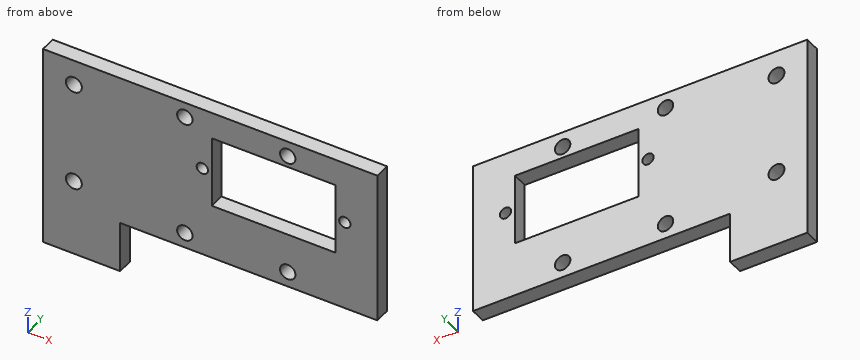
```python
from build123d import *

# Parameters (mm, degrees)
SKETCH_1_W          = 65
SKETCH_1_H          = 40
EXTRUDE_1_DEPTH     = 3
SKETCH_2_R          = 1.55
CUT_EXTRUDE_1_DEPTH = 10
SKETCH_3_W          = 50
SKETCH_3_H          = 10
CUT_EXTRUDE_2_DEPTH = 10
SKETCH_4_W          = 24
SKETCH_4_H          = 14
CUT_EXTRUDE_3_DEPTH = 10
SKETCH_5_R          = 1.1
CUT_EXTRUDE_4_DEPTH = 10
SKETCH_6_R          = 1.5
CUT_EXTRUDE_5_DEPTH = 25


with BuildPart() as part:
    # 草图1 → 凸台-拉伸1 (new body)
    with BuildSketch(Plane(origin=(0, 0, 0), x_dir=(1, 0, 0), z_dir=(0, 1, 0))):
        Rectangle(SKETCH_1_W, SKETCH_1_H)
    extrude(amount=EXTRUDE_1_DEPTH)

    # 草图2 → 切除-拉伸1 (cut)
    with BuildSketch(Plane(origin=(0, 0, 0), x_dir=(-1, 0, 0), z_dir=(0, -1, 0))):
        with Locations(Location((26.5, -15, 0), (0, 0, 90))):
            Circle(SKETCH_2_R)
        with Locations(Location((26.5, 5, 0), (0, 0, 90))):
            Circle(SKETCH_2_R)
    extrude(amount=-CUT_EXTRUDE_1_DEPTH, mode=Mode.SUBTRACT)

    # 草图3 → 切除-拉伸2 (cut)
    with BuildSketch(Plane(origin=(0, 0, 0), x_dir=(-1, 0, 0), z_dir=(0, -1, 0))):
        with Locations((-7.5, 15)):
            Rectangle(SKETCH_3_W, SKETCH_3_H)
    extrude(amount=-CUT_EXTRUDE_2_DEPTH, mode=Mode.SUBTRACT)

    # 草图4 → 切除-拉伸3 (cut)
    with BuildSketch(Plane(origin=(0, 0, 0), x_dir=(-1, 0, 0), z_dir=(0, -1, 0))):
        with Locations((-12.32495, -7.75)):
            Rectangle(SKETCH_4_W, SKETCH_4_H)
    extrude(amount=-CUT_EXTRUDE_3_DEPTH, mode=Mode.SUBTRACT)

    # 草图5 → 切除-拉伸4 (cut)
    with BuildSketch(Plane(origin=(0, 3, 0), x_dir=(1, 0, 0), z_dir=(0, 1, 0))):
        with Locations(Location((26.17495, -7.75, 0), (0, 0, 270))):
            Circle(SKETCH_5_R)
        with Locations(Location((-1.52505, -7.75, 0), (0, 0, 270))):
            Circle(SKETCH_5_R)
    extrude(amount=-CUT_EXTRUDE_4_DEPTH, mode=Mode.SUBTRACT)

    # 草图6 → 切除-拉伸5 (cut)
    with BuildSketch(Plane(origin=(0, 0, 0), x_dir=(-1, 0, 0), z_dir=(0, -1, 0))):
        with Locations(Location((-15.074975, -17, 0), (0, 0, 90))):
            Circle(SKETCH_6_R)
        with Locations(Location((4.925025, -17, 0), (0, 0, 90))):
            Circle(SKETCH_6_R)
        with Locations(Location((-15.074975, 7, 0), (0, 0, 90))):
            Circle(SKETCH_6_R)
        with Locations(Location((4.925025, 7, 0), (0, 0, 90))):
            Circle(SKETCH_6_R)
    extrude(amount=-CUT_EXTRUDE_5_DEPTH, mode=Mode.SUBTRACT)


solid = part.part
```
Input: part model. Units: mm. Frame: model coordinates. Coordinates: 2 decimals unless noted, no trailing zeros. Loops run counter-clockwise (first coordinate to the right, second up) from the corner with the lowest first, then second, coordinate; pieces in that order, holes last. Notation, with made-up numbers: M -38,84 L -32,84 A15 ccw -32,90 Z; hole C 21,-16 d11. An arc over 180 degrees is marked long. Use a Markdown table: item, result. Add a question column.
1) Line query: L1, parallel to X at y = 1.25, z = 7.75; L2, parallel to X at y = 1.5, z = -5; L3, parallel to X at y = 0.65, z = 13. Output: solid intervals per line, ascending. Write a range as from..to.
2) Section C-C, the plane x = -26.5. Return the cut outline in (y, z).
3) Section D-D, the plane z = 7.75. Return the cut outline in (x, y).
4) Section B-B, the plane z = 12.5. Return the cut outline in (x, y).
5) Pin query (flat end, axial travel): P1, Ø1.5, axis at x = 15.5, y = 0.5, coming from the -Z side; P2, Ø4, axis at x = 11, z = 12, coming from the +Y side; P3, Ø0.9, axis at y = 1.5, z = -13, coming from the +X side. Return the tip coordinate at first contact, or that it passes through.
6) Section A-A, the plane x = 9. Return the cut outline in (y, z), plus the area to 3 significant figures.
Answer below:
| question | item | result |
|---|---|---|
| 1 | L1 | -32.5..-2.63, -0.43..0.32, 24.32..25.07, 27.27..32.5 |
| 1 | L2 | -32.5..-28.05, -24.95..32.5 |
| 1 | L3 | -32.5..0.32, 24.32..32.5 |
| 2 | outline | M 0,-20 L 3,-20 L 3,-6.55 L 0,-6.55 Z; M 0,-3.45 L 3,-3.45 L 3,13.45 L 0,13.45 Z; M 0,16.55 L 3,16.55 L 3,20 L 0,20 Z |
| 3 | outline | M -32.5,0 L -2.63,0 L -2.63,3 L -32.5,3 Z; M -0.43,0 L 0.32,0 L 0.32,3 L -0.43,3 Z; M 24.32,0 L 25.07,0 L 25.07,3 L 24.32,3 Z; M 27.27,0 L 32.5,0 L 32.5,3 L 27.27,3 Z |
| 4 | outline | M -32.5,0 L 0.32,0 L 0.32,3 L -32.5,3 Z; M 24.32,0 L 32.5,0 L 32.5,3 L 24.32,3 Z |
| 5 | P1 | z = -10 |
| 5 | P2 | through |
| 5 | P3 | x = -17.5 |
| 6 | outline | M 0,-10 L 3,-10 L 3,0.75 L 0,0.75 Z; M 0,14.75 L 3,14.75 L 3,20 L 0,20 Z |
| 6 | area | 48.0 mm2 |
